Could you check a few things on this drawing? It's one solid part, dimensions in mm from its lowest x, y, z. A direction names the side the tool comes from. Round coordinates to 2 decimals unless told otherwise and drop trailing zeros. Use a Markdown table: item, result. Add a question column.
(1) Thinking about a two-plate mould opening in X: for the marked faces 4, 5, 6 and 7, which applies, pulls with the +X half, pulls with the -X half, needs draft (parallel to the pull), parting line crosses it, or undercut?
(2) I'm going to push flat-ended pins straight in: P1, Ø10, axis at y = 26.5, z = 28, coming from the +X side; P2, Ø10, axis at x = 16, y = 8, coming from the -Z side; P3, Ø19, axis at x = 20.5, z = 12.5, coming from the +Y side; P4, Ø3, axis at x = 20, z = 24, coming from the +Y side. Where does each tip first touch, or does it pass through?
(3) If I drill on probe 1 along Z at (x, y) = (19, 2) (1 decimal); probe 2 along Y at (x, z) = (17.5, 6.5); probe 3 along X at (y, z) = (32, 31.5) (1 decimal), over which ranges is the centre line in solid material (lowest first)?
(4) On a 3-axis mill with a long thin cutter (end or side, diameter ignored), from which of +Z, -Z, +X, -X, +Y, -Y can I reach the whole of each face in a straight line? I mean the marked faces 1, 2 and 3. Say none if no direction works.
(5) I want a section at C-C, the plane z = 14. Give the number of separate pieces and of enclosed holes in the cut face, then the cut area to 3 significant figures.
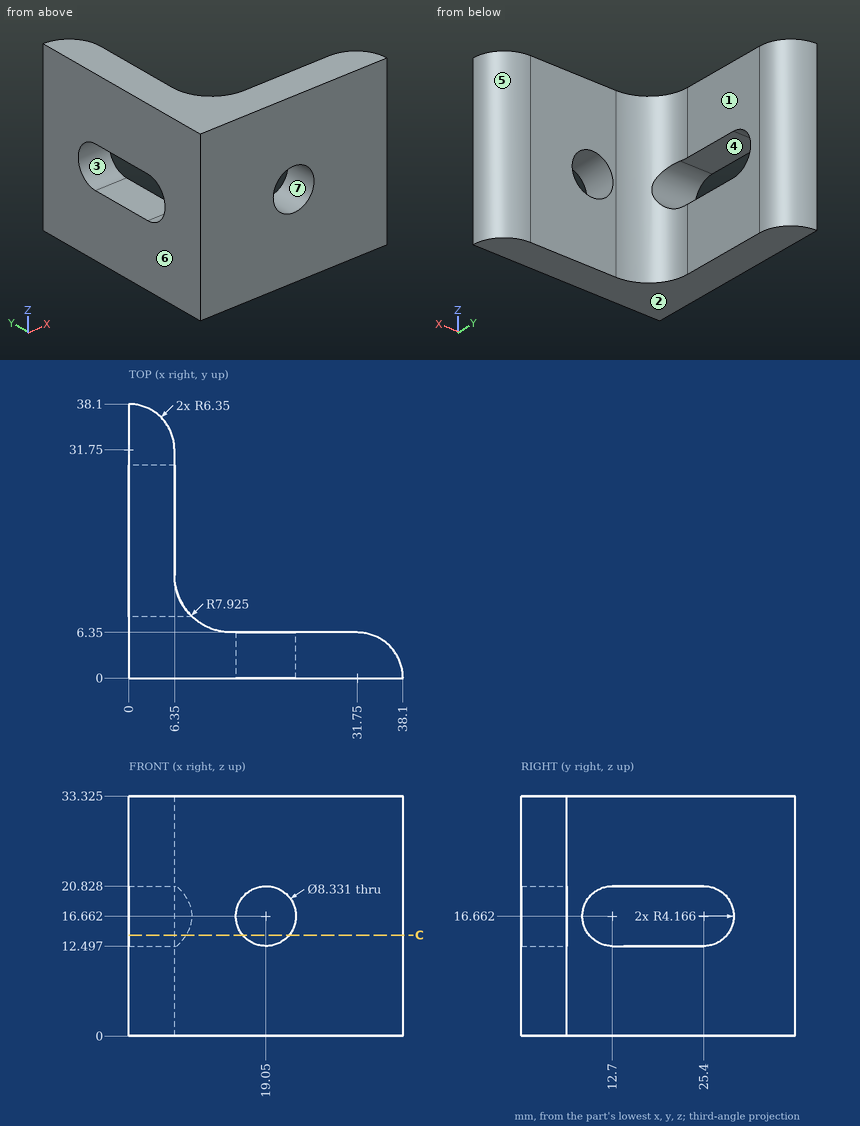
Taken from the geometry:
| question | item | result |
|---|---|---|
| 1 | face 4 | needs draft |
| 1 | face 5 | pulls with the +X half |
| 1 | face 6 | pulls with the -X half |
| 1 | face 7 | undercut |
| 2 | P1 | stops at x = 6.35 |
| 2 | P2 | stops at z = 0 |
| 2 | P3 | stops at y = 7.06 |
| 2 | P4 | stops at y = 6.35 |
| 3 | probe 1 | z = 0 to 12.5, 20.8 to 33.3 |
| 3 | probe 2 | y = 0 to 6.35 |
| 3 | probe 3 | x = 0 to 6.3 |
| 4 | face 1 | +Z, -Z, +X, +Y |
| 4 | face 2 | -Z, +X, -X, +Y, -Y |
| 4 | face 3 | +X, -X |
| 5 | separate pieces | 3 |
| 5 | enclosed holes | 0 |
| 5 | area | 275 mm2 |
